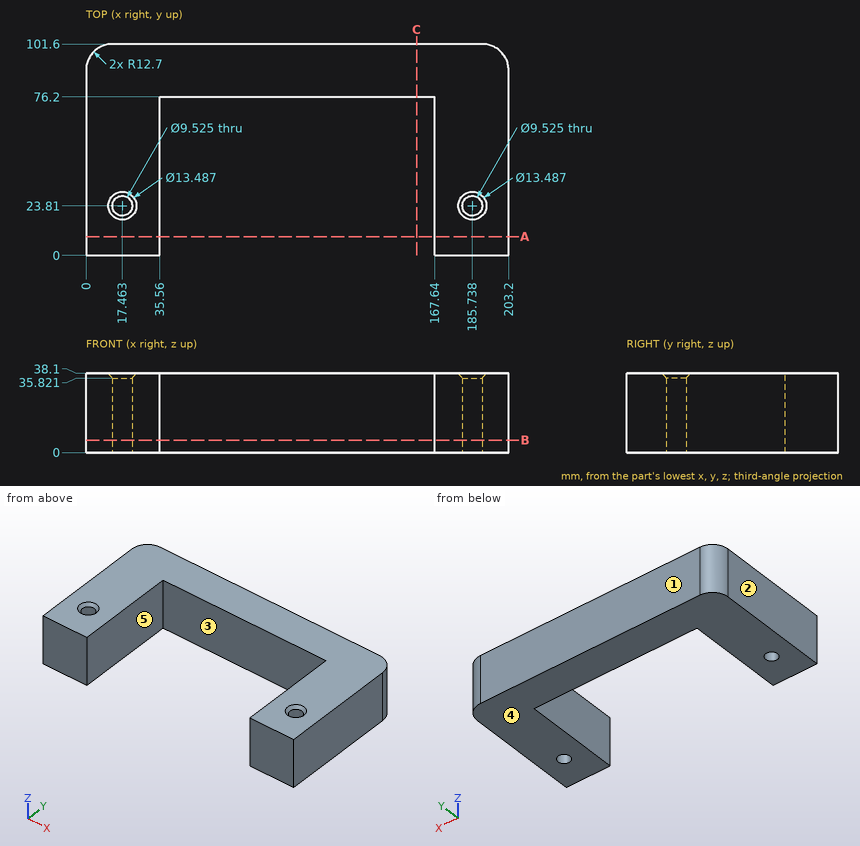
Answer from the drawing. Dimensions are ordinates in mm from the lowest x, y and z of the part. A direction names the side the tool comes from. Coordinates: 2 decimals unless noted, no trailing zeros. Write each loop counter-clockwise with the first axis right and the second up, starting at its lowest first coordinate (ties: lowest second). Pieces come first, ordered by that corner, then holes. Notation, with made-up numbers: (59.5, 30.5) - (89.5, 30.5) arc R32 cw to (89.5, 67.5) - close; hole circle Ø9 at (76, 49). An arc over 180 degrees is marked (long way). Return JSON: item names as keys, results as strings. Group by question number.
Q1. Which of the six approach directions +Z, -Z, +X, -X, +Y, -Y give full straight-line access (tool end or side, diameter ignored) to the marked faces 4 and 5?
Q2. The part is cut by section C-C on x = 159. Write down the section's boundary in (y, z), and give its area (3 significant figures).
Q3. For a pull along X with two mould halves and no side action, classify the marked faces 1, 2 and 3 as +X half, -X half, draft (parallel to the pull), parting line (faces both ways), or undercut.
Q4. The part is cut by section A-A on y = 9. Write down the section's boundary in (x, z).
Q5. Find the intervals of material crossed by line 1 along X through (y, z) = (57.5, 13); line 2 along X through (y, z) = (26, 19) (1 decimal); line 3 along Y through (x, z) = (87, 17), in increasing order. Write a range as [from, to].
Q6. Flat-ended cylindrical pins translate along their axes: pin 1 Ø11 at (x, y) = (17.46, 23.81) entering from +Z; pin 2 Ø19 at (x, z) = (98, 24) entering from -Y; pin 3 Ø12 at (x, y) = (72.5, 64.5) entering from -Z. Find the tip coordinate at first contact, or state that the pin passes through.
Q7. The part is cut by section B-B on z = 6. Write down the section's boundary in (x, y) (1 decimal), and give its area (3 significant figures).
Evaluation:
{
 "1": {"face 4": "-Z, +X, -X, +Y, -Y", "face 5": "+Z, -Z, -Y"},
 "2": {"outline": "(76.2, 0) - (101.6, 0) - (101.6, 38.1) - (76.2, 38.1) - close", "area": "968 mm2"},
 "3": {"face 1": "draft", "face 2": "-X half", "face 3": "undercut"},
 "4": {"outline": "(0, 0) - (35.56, 0) - (35.56, 38.1) - (0, 38.1) - close; (167.64, 0) - (203.2, 0) - (203.2, 38.1) - (167.64, 38.1) - close"},
 "5": {"line 1": "x = [0, 35.56], [167.64, 203.2]", "line 2": "x = [0, 13.2], [21.7, 35.6], [167.6, 181.5], [190, 203.2]", "line 3": "y = [76.2, 101.6]"},
 "6": {"pin 1": "stops at z = 36.67", "pin 2": "stops at y = 76.2", "pin 3": "passes through"},
 "7": {"outline": "(0, 0) - (35.6, 0) - (35.6, 76.2) - (167.6, 76.2) - (167.6, 0) - (203.2, 0) - (203.2, 88.9) arc R12.7 ccw to (190.5, 101.6) - (12.7, 101.6) arc R12.7 ccw to (0, 88.9) - close; hole circle Ø9.5 at (17.5, 23.8); hole circle Ø9.5 at (185.7, 23.8)", "area": "10,400 mm2"}
}
